Read the model definition and answer for the solid it produces. Units are mm, in the model's axes. A direction names the side the tool comes from. Give positions to 0.01 mm unless a question says otherwise; leave off trailing zeros. Order: outer loops, then holes, each group sorted by start corner. A loop starts at its lowest first (then second) coordinate and runs counter-clockwise, first axis right, second up. Notation, with made-up numbers: (-32.5, 42.25) - (10.5, 42.25) arc R26 ccw to (10.5, 70.25) - close; hole circle Ø11 at (-2, 23.5). An arc over 180 degrees is marked (long way). Use a Markdown table: item, result. Add a question column.
1. A cutting plane is placed at A-A on y = 0. Determine the outline of the cut face in (x, z).
2. For a pull along Y with two mould halves and no side action, classify faces 1 (the cylindrical face through (3.16, 1, -0.09)), 2 (the flat face through (16, -8, -6.35)), 3 (the flat face through (16, 4.667, 9)) as released by +Y, released by -Y, zero draft, split by the parting line, or undercut.
3. A cutting plane is placed at B-B on x = 38.1. Determine the outline of the cut face in (y, z).
4. Consider L1, parallel to Y at x = 0, z = -2; L2, parallel to Y at x = -1, z = -9.5; L3, parallel to Z at x = 43.5, y = -7. Determine where each line is inside the solid, lowest interval first.
5. A cutting plane is placed at D-D on x = -9. Determine the outline of the cut face in (y, z).
6. Flat-ended cylindrical pins translate along their axes: P1, Ø10, axis at x = 44.5, y = -13.5, coming from the -Z side; P2, Ø4, axis at y = -5, z = 0.5, coming from the +X side; P3, Ø10, axis at x = -8.5, z = -15, coming from the -Y side. Find the tip coordinate at first contact, or state that the pin passes through.
7. Which of the six approach directions +Z, -Z, +X, -X, +Y, -Y give full straight-line access (tool end or side, diameter ignored) to faces 4 (the flat face through (-13.672, -8, 0)), 5 (the flat face through (47.44, -8, 0)), 6 (the flat face through (16, -8, 6.35)), 7 (the flat face through (16, 10, 19.05)), 8 (the flat face through (16, 14.827, 0))?
8. A cutting plane is placed at C-C on z = -4. Determine the outline of the cut face in (x, y), and give its area (3 significant figures).
```python
from build123d import *

# Parameters (mm, degrees)
SKETCH2_W           = 61.111815401
SKETCH2_H           = 25.256192137
SKETCH2_R           = 3.313116642
BOSS_EXTRUDE6_DEPTH = 6.35
SKETCH2_5_W         = 76.588209157
SKETCH2_5_H         = 10.16
BOSS_EXTRUDE7_DEPTH = 19.05


with BuildPart() as part:
    # Sketch2 → Boss-Extrude6 (new, symmetric)
    with BuildSketch(Plane.XY):
        with Locations((16.884167922, -7.961511284)):
            Rectangle(SKETCH2_W, SKETCH2_H)
        Circle(SKETCH2_R, mode=Mode.SUBTRACT)
        with Locations((38.1, 0)):
            Circle(SKETCH2_R, mode=Mode.SUBTRACT)
    extrude(amount=BOSS_EXTRUDE6_DEPTH, both=True)

    # Sketch2<5> → Boss-Extrude7 (add, symmetric)
    with BuildSketch(Plane.XY):
        with Locations((16.624239124, 9.746584785)):
            Rectangle(SKETCH2_5_W, SKETCH2_5_H)
    extrude(amount=BOSS_EXTRUDE7_DEPTH, both=True)


solid = part.part
```
Output values:
| question | item | result |
|---|---|---|
| 1 | outline | (-13.67, -6.35) - (-3.31, -6.35) - (-3.31, 6.35) - (-13.67, 6.35) - close; (3.31, -6.35) - (34.79, -6.35) - (34.79, 6.35) - (3.31, 6.35) - close; (41.41, -6.35) - (47.44, -6.35) - (47.44, 6.35) - (41.41, 6.35) - close |
| 2 | face 1 | undercut |
| 2 | face 2 | zero draft |
| 2 | face 3 | released by -Y |
| 3 | outline | (-20.59, -6.35) - (-3.31, -6.35) - (-3.31, 6.35) - (-20.59, 6.35) - close; (3.31, -6.35) - (4.67, -6.35) - (4.67, -19.05) - (14.83, -19.05) - (14.83, 19.05) - (4.67, 19.05) - (4.67, 6.35) - (3.31, 6.35) - close |
| 4 | L1 | -20.59 to -3.31, 3.31 to 14.83 |
| 4 | L2 | 4.67 to 14.83 |
| 4 | L3 | -6.35 to 6.35 |
| 5 | outline | (-20.59, -6.35) - (4.67, -6.35) - (4.67, -19.05) - (14.83, -19.05) - (14.83, 19.05) - (4.67, 19.05) - (4.67, 6.35) - (-20.59, 6.35) - close |
| 6 | P1 | z = -6.35 |
| 6 | P2 | x = 47.44 |
| 6 | P3 | y = 4.67 |
| 7 | face 4 | +Z, -Z, -X, -Y |
| 7 | face 5 | +Z, -Z, +X, -Y |
| 7 | face 6 | +Z, +X, -X, -Y |
| 7 | face 7 | +Z, +X, -X, +Y, -Y |
| 7 | face 8 | +Z, -Z, +X, -X, +Y |
| 8 | outline | (-21.67, 4.67) - (-13.67, 4.67) - (-13.67, -20.59) - (47.44, -20.59) - (47.44, 4.67) - (54.92, 4.67) - (54.92, 14.83) - (-21.67, 14.83) - close; hole circle Ø6.63 at (0, 0); hole circle Ø6.63 at (38.1, 0) |
| 8 | area | 2,250 mm² |
